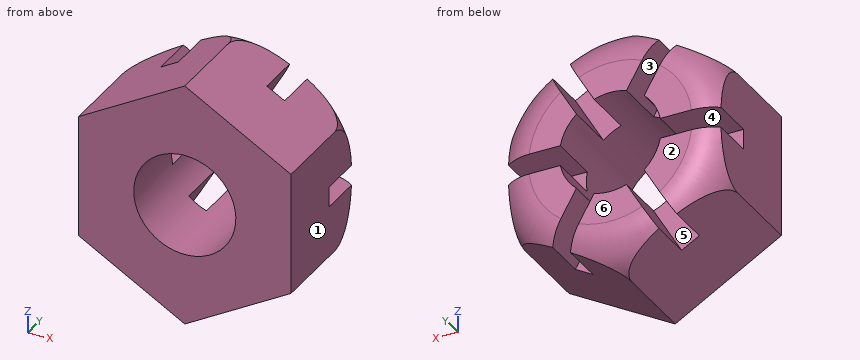
```python
from build123d import *

# Parameters (mm, degrees)
BOSS_EXTRUDE1_DEPTH = 15.24
CUT_EXTRUDE2_DEPTH  = 6.35
SKETCH8_R           = 6.35
CUT_EXTRUDE4_DEPTH  = 26.284591317


with BuildPart() as part:
    # Sketch1 → Boss-Extrude1 (new body)
    with BuildSketch(Plane(origin=(0, 0, 0), x_dir=(1, 0, 0), z_dir=(0, 1, 0))):
        Polygon((0, 15.251284711), (-13.208, 7.625642355), (-13.208, -7.625642355), (0, -15.251284711), (13.208, -7.625642355), (13.208, 7.625642355), align=None)
    extrude(amount=BOSS_EXTRUDE1_DEPTH)

    # Sketch2 → Cut-Revolve2 (revolve, cut)
    with BuildSketch(Plane(origin=(0, 0, 0), x_dir=(0, 0, -1), z_dir=(1, 0, 0))):
        with BuildLine():
            Line((15.251284711, 10.16), (15.251284711, 0))
            Line((15.251284711, 0), (20.607145121, 0))
            Line((20.607145121, 0), (20.607145121, 19.004731249))
            Line((20.607145121, 19.004731249), (7.625642355, 19.004731249))
            Line((7.625642355, 19.004731249), (7.625642355, 15.24))
            Line((7.625642355, 15.24), (10.171284711, 15.24))
            ThreePointArc((10.171284711, 15.24), (13.763387159, 13.752102448), (15.251284711, 10.16))
        make_face()
    revolve(axis=Axis((0, 0, 0), (0, 1, 0)), mode=Mode.SUBTRACT)

    # Sketch4 → Cut-Extrude2 (cut)
    with BuildSketch(Plane(origin=(0, 15.24, 0), x_dir=(1, 0, 0), z_dir=(0, 1, 0))):
        Polygon((-7.703852263, 10.803463533), (-2.199704526, 1.27), (-13.208, 1.27), (-13.208, -1.27), (-2.199704526, -1.27), (-7.703852263, -10.803463533), (-5.504147737, -12.073463533), (0, -2.54), (5.504147737, -12.073463533), (7.703852263, -10.803463533), (2.199704526, -1.27), (13.208, -1.27), (13.208, 1.27), (2.199704526, 1.27), (7.703852263, 10.803463533), (5.504147737, 12.073463533), (0, 2.54), (-5.504147737, 12.073463533), align=None)
    extrude(amount=-CUT_EXTRUDE2_DEPTH, mode=Mode.SUBTRACT)

    # Sketch8 → Cut-Extrude4 (cut, through all)
    with BuildSketch(Plane(origin=(0, 15.24, 0), x_dir=(1, 0, 0), z_dir=(0, 1, 0))):
        with Locations(Location((0, 0, 0), (0, 0, 270))):
            Circle(SKETCH8_R)
    extrude(amount=-CUT_EXTRUDE4_DEPTH, mode=Mode.SUBTRACT)


solid = part.part
```
Geometry check sheet. Reference: the model listing, model coordinates, mm. Face numbers are marked on the shaded views. A direction names the side the tool comes from. Coordinates: 2 decimals unless noted, no trailing zeros. Order: outer loops, then holes, each group sorted by start corner. A loop starts at its lowest first (then second) coordinate and runs counter-clockwise, first axis right, second up. Notation, with made-up numbers: (-32.75, 38) - (-23.75, 38) arc R20 ccw to (-23.75, 46) - close; hole circle Ø5 at (42, 81.25). An arc over 180 degrees is marked (long way). Use one line per item in the form item = value.
1. Section check C-C (y = 13.5). State how many separate pieces and enclosed holes the cut face has, then the cut area to 3 significant figures.
Here are the results:
separate_pieces = 6
enclosed_holes = 0
area = 354 mm²
2. Section check B-B (z = 0). Record the boundary of the cut face in (x, y).
Here are the results:
outline = (-13.21, 0) - (-6.35, 0) - (-6.35, 8.89) - (-13.21, 8.89) - close; (6.35, 0) - (13.21, 0) - (13.21, 8.89) - (6.35, 8.89) - close
3. Draft check along X on the marked faces 1, 2 and 3. Enter one of: pulls with the +X half, pulls with the -X half, needs draft (parallel to the pull), parting line crosses it, or undercut.
Here are the results:
face_1 = pulls with the +X half
face_2 = needs draft
face_3 = undercut
4. Access from +Z, -Z, +X, -X, +Y, -Y to the whole of each face (thin tool, end or side, straight path). Record for the marked faces 4, 5 and 6.
Here are the results:
face_4 = +X, -X, +Y
face_5 = +Y
face_6 = +Z, -Z, +X, -X, +Y
5. Scan lines: line 1 (Z direction, x = 0, y = 7.5); line 2 (X direction, y = 6.75, z = 0); line 3 (X direction, y = 11, z = -8). Record each from-to range of solid material in increasing order.
Here are the results:
line_1 = -15.25 to -6.35, 6.35 to 15.25
line_2 = -13.21 to -6.35, 6.35 to 13.21
line_3 = -12.56 to -6.09, -3.15 to 3.15, 6.09 to 12.56
6. Gauge pin test, flat ends, axial feed: pin 1 (3 mm diameter, centred on x = 2.5, y = 8.5, fed in from -Z); pin 2 (4.5 mm diameter, centred on x = -5, z = -9, fed in from +Y); pin 3 (1.7 mm diameter, centred on x = 5, z = 8.5, fed in from +Y); pin 4 (1.9 mm diameter, centred on x = -10.5, y = 13, fed in from -Z). Record the tip position at first contact, or that the pin passes through.
Here are the results:
pin_1 = -14.67
pin_2 = 15.24
pin_3 = 8.89
pin_4 = -9.74
7. Section check A-A (y = 4.75). Record the boundary of the cut face in (x, z), then the cut area to 3 significant figures.
Here are the results:
outline = (-13.21, -7.63) - (0, -15.25) - (13.21, -7.63) - (13.21, 7.63) - (0, 15.25) - (-13.21, 7.63) - close; hole circle Ø12.7 at (0, 0)
area = 478 mm²
